from build123d import *

# Parameters (mm, degrees)
BOSS_EXTRUDE1_DEPTH = 15
SKETCH2_R           = 1.7
CUT_EXTRUDE1_DEPTH  = 35.655960635
CUT_EXTRUDE2_DEPTH  = 6.066365529
CUT_EXTRUDE3_REACH  = 36.656
SKETCH4_R           = 1.35
CUT_EXTRUDE4_REACH  = 36.656
SKETCH5_R           = 1.350000001
CHAMFER2_SIZE       = 9
CHAMFER2_SIZE2      = 5.196152423


with BuildPart() as part:
    # Sketch1 → Boss-Extrude1 (new body)
    with BuildSketch(Plane.XY):
        with BuildLine():
            Line((0, 0), (20, 0))
            Line((20, 0), (20, 9.066365529))
            Line((20, 9.066365529), (8, 9.066365529))
            Line((8, 9.066365529), (5, 9.066365529))
            ThreePointArc((5, 9.066365529), (2.066666667, 11.999698862), (5, 14.933032196))
            Line((5, 14.933032196), (12.6, 14.933032196))
            ThreePointArc((12.6, 14.933032196), (16.118831006, 16.608004693), (17.03761247, 20.395292))
            ThreePointArc((17.03761247, 20.395292), (17.240267675, 21.230652218), (18.016414611, 21.600100131))
            Line((18.016414611, 21.600100131), (20, 21.600100131))
            Line((20, 21.600100131), (20, 24.000741841))
            Line((20, 24.000741841), (0, 24))
            Line((0, 24), (0, 22.4))
            Line((0, 22.4), (12.6, 22.4))
            ThreePointArc((12.6, 22.4), (15.533250224, 19.466749776), (12.6, 16.533499552))
            Line((12.6, 16.533499552), (5, 16.533499552))
            ThreePointArc((5, 16.533499552), (0.46628242, 11.999781972), (5, 7.466064391))
            Line((5, 7.466064391), (8, 7.466064391))
            ThreePointArc((8, 7.466064391), (10.933032196, 4.533032196), (8, 1.6))
            Line((8, 1.6), (0, 1.6))
            Line((0, 1.6), (0, 0))
        make_face()
    extrude(amount=BOSS_EXTRUDE1_DEPTH)

    # Sketch2 → Cut-Extrude1 (cut, through all)
    with BuildSketch(Plane(origin=(-0.000890209, 23.999999967, 0), x_dir=(0.9999999993120905, 3.709203365043046e-05, 0), z_dir=(-3.709203365043046e-05, 0.9999999993120905, 0))):
        with Locations(Location((16.000890209, -7.5, 0), (0, 0, 180))):
            Circle(SKETCH2_R)
    extrude(amount=-CUT_EXTRUDE1_DEPTH, mode=Mode.SUBTRACT)

    # Sketch3 → Cut-Extrude2 (cut)
    with BuildSketch(Plane.XZ):
        Polygon((21.085370845, -1.090112753), (21.085370845, 10.848631561), (16.00089022, 10.848631561), (13.10089022, 9.174315781), (13.10089022, -1.090112753), align=None)
    extrude(amount=-CUT_EXTRUDE2_DEPTH, mode=Mode.SUBTRACT)

    # Sketch4 → Cut-Extrude3 (cut, up to next)
    with BuildSketch(Plane(origin=(-0.000890209, 23.999999967, 0), x_dir=(0.9999999993120905, 3.709203365043046e-05, 0), z_dir=(-3.709203365043046e-05, 0.9999999993120905, 0)), mode=Mode.PRIVATE) as cut_extrude3_sk1:
        with Locations(Location((3.000890209, -7.5, 0), (0, 0, 180))):
            Circle(SKETCH4_R)
    cut_extrude3_tool1 = extrude(cut_extrude3_sk1.sketch, amount=-CUT_EXTRUDE3_REACH, mode=Mode.PRIVATE) & part.part
    add(cut_extrude3_tool1.solids().sort_by_distance((3, 24.000111, 7.5))[0], mode=Mode.SUBTRACT)

    # Sketch5 → Cut-Extrude4 (cut, up to next)
    with BuildSketch(Plane.XZ, mode=Mode.PRIVATE) as cut_extrude4_sk1:
        with Locations(Location((3.000059349, 7.5, 0), (0, 0, 270))):
            Circle(SKETCH5_R)
    cut_extrude4_tool1 = extrude(cut_extrude4_sk1.sketch, amount=-CUT_EXTRUDE4_REACH, mode=Mode.PRIVATE) & part.part
    add(cut_extrude4_tool1.solids().sort_by_distance((3.000059, 0, 7.5))[0], mode=Mode.SUBTRACT)

    # Chamfer2
    chamfer2_edges = [part.edges().sort_by_distance(p)[0] for p in [
        (20, 7.566365529, 0),
    ]]
    chamfer2_side = [part.faces().sort_by_distance(p)[0] for p in [
        (0.778698106, 11.999781972, 0),
    ]]
    chamfer(chamfer2_edges, length=CHAMFER2_SIZE, length2=CHAMFER2_SIZE2, reference=chamfer2_side[0])


solid = part.part
Geometry check sheet. Reference: the model listing, model coordinates, mm. A direction names the side the tool comes from. Give positions to 0.01 mm unless a question says otherwise; leave off trailing zeros. Order: outer loops, then holes, each group sorted by start corner. A loop starts at its lowest first (then second) coordinate and runs counter-clockwise, first axis right, second up. Notation, with made-up numbers: (-20.75, 42) - (13.25, 42) arc R19 ccw to (13.25, 74) - close; hole circle Ø9 at (40, -18.75). An arc over 180 degrees is marked (long way). Answer as a JSON object with one key per item and string values.
(1) Depth check by flat-ended pin: pin 1 Ø2 at (y, z) = (12, 8) entering from -X; pin 2 Ø1.5 at (y, z) = (7.5, 8) entering from -X; pin 3 Ø1.6 at (x, z) = (3, 7.5) entering from -Y. Enter the tip coordinate at first touch or a pass-through.
Report:
{"pin 1": "x = 0.47", "pin 2": "x = 2.45", "pin 3": "y = 7.63"}
(2) Cross-section at A-A (x = 5.5). Record the cut outline in (y, z).
Report:
{"outline": "(0, 0) - (1.6, 0) - (1.6, 15) - (0, 15) - close; (7.47, 0) - (9.07, 0) - (9.07, 15) - (7.47, 15) - close; (14.93, 0) - (16.53, 0) - (16.53, 15) - (14.93, 15) - close; (22.4, 0) - (24, 0) - (24, 15) - (22.4, 15) - close"}
(3) Material ranges on line 1 (X direction, y = 23.65, z = 7.5); line 2 (X direction, y = 0.75, z = 7.5); line 3 (Y direction, x = 18.5, z = 14), recorded low to high.
Report:
{"line 1": "0 to 1.65, 4.35 to 14.3, 17.7 to 20", "line 2": "0 to 1.65, 4.35 to 13.1", "line 3": "0 to 9.07, 21.6 to 24"}
(4) Draft check along Y on faces 1 (the cylindrical face through (17.23, 21.22, 5.73)), 2 (the flat face through (14.571, 2.991, 10.023)), 3 (the flat face through (5, 1.6, 7)). Enter one of: released by +Y, released by -Y, zero draft, split by the parting line, or undercut.
Report:
{"face 1": "undercut", "face 2": "zero draft", "face 3": "undercut"}
(5) Cross-section at C-C (x = 11.5). Record the cut outline in (y, z).
Report:
{"outline": "(0, 0.29) - (9.07, 0.29) - (9.07, 15) - (0, 15) - close; (14.93, 0) - (16.53, 0) - (16.53, 15) - (14.93, 15) - close; (22.4, 0) - (24, 0) - (24, 15) - (22.4, 15) - close"}
(6) Tool access check on faces 4 (the flat face through (20, 23, 7)), 5 (the flat face through (9, 16.533, 7)), 6 (the flat face through (8, 16, 0)), 7 (the flat face through (19, 21.6, 7)). Record the directions out of +Z, -Z, +X, -X, +Y, -Y that give a thin tool (end or side, any length) a straight path to the whole face; none if there is none.
Report:
{"face 4": "+Z, -Z, +X, +Y, -Y", "face 5": "+Z, -Z, -X", "face 6": "-Z, +X, -X, +Y, -Y", "face 7": "+Z, -Z, +X"}
(7) Cross-section at D-D (y = 3). Record the cut outline in (x, z), then the cut area to 3 significant figures.
Report:
{"outline": "(10.5, 0) - (11, 0) - (13.1, 1.21) - (13.1, 9.17) - (16, 10.85) - (20, 10.85) - (20, 15) - (10.5, 15) - close", "area": "68.8 mm^2"}
(8) Cross-section at B-B (z = 2.75). Record the cut outline in (x, y), then the cut area to 3 significant figures.
Report:
{"outline": "(0, 0) - (13.1, 0) - (13.1, 6.07) - (15.76, 6.07) - (15.76, 9.07) - (5, 9.07) arc R2.93 cw to (5, 14.93) - (12.6, 14.93) arc R4.53 ccw to (17.04, 20.4) arc R1 cw to (18.02, 21.6) - (20, 21.6) - (20, 24) - (0, 24) - (0, 22.4) - (12.6, 22.4) arc R2.93 cw to (12.6, 16.53) - (5, 16.53) arc R4.53 ccw to (5, 7.47) - (8, 7.47) arc R2.93 cw to (8, 1.6) - (0, 1.6) - close", "area": "140 mm^2"}
